Input: dimensioned drawing with shaded views. Units: mm. Origin: part minimum x, y, z. A direction names the side the tool comes from. Coordinates: 2 decimals unless noted, no trailing zeros. Write each loop counter-clockwise with the first axis right and the second up, starting at its lowest first coordinate (ties: lowest second). Pieces come first, ordered by that corner, then holes. Notation, with made-up numbers: M 19.5,68 L 49.5,68 A13 ccw 49.5,93 Z; hole C 23,19 d7. An arc over 180 degrees is marked long. Use one line per item in the form item = value.
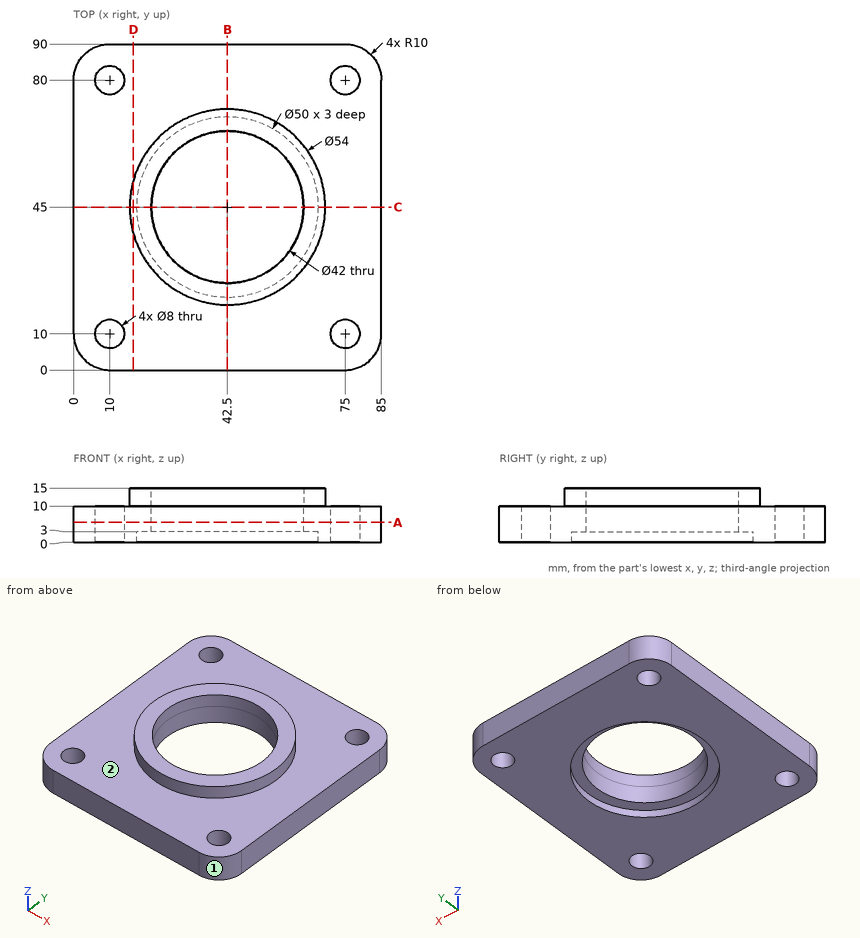
(1) Section query C-C on y = 45. Return the cut outline in (x, z), plus the area to 3 significant figures.
Computed:
outline = M 0,0 L 17.5,0 L 17.5,3 L 21.5,3 L 21.5,15 L 15.5,15 L 15.5,10 L 0,10 Z; M 63.5,3 L 67.5,3 L 67.5,0 L 85,0 L 85,10 L 69.5,10 L 69.5,15 L 63.5,15 Z
area = 466 mm^2
(2) Section query A-A on z = 5.5. Return the cut outline in (x, y), plus the area to 3 significant figures.
Computed:
outline = M 0,10 A10 ccw 10,0 L 75,0 A10 ccw 85,10 L 85,80 A10 ccw 75,90 L 10,90 A10 ccw 0,80 Z; hole C 10,10 d8; hole C 10,80 d8; hole C 42.5,45 d42; hole C 75,10 d8; hole C 75,80 d8
area = 5,980 mm^2
(3) Set-up query: the marked faces 1 and 2. Return all of +Z, -Z, +X, -X, +Y, -Y with unobstructed straight access to the full face (end or side cutting, diameter ignored); none if empty.
Computed:
face_1 = +Z, -Z, +X, -Y
face_2 = +Z
(4) Section query B-B on x = 42.5. Return the cut outline in (y, z), plus the area to 3 significant figures.
Computed:
outline = M 0,0 L 20,0 L 20,3 L 24,3 L 24,15 L 18,15 L 18,10 L 0,10 Z; M 66,3 L 70,3 L 70,0 L 90,0 L 90,10 L 72,10 L 72,15 L 66,15 Z
area = 516 mm^2
(5) First-contact query: pin 1 Ø1.5 at (x, z) = (20, 12) entering from +Y; pin 2 Ø1 at (x, z) = (64.5, 12) entering from -Y. Flat tips, straight axial feed; report the tip coordinate or a pass-through.
Computed:
pin_1 = 61
pin_2 = 28.67
(6) Section query D-D on x = 16.5. Return the cut outline in (y, z), plus the area to 3 significant figures.
Computed:
outline = M 0,0 L 90,0 L 90,10 L 52.28,10 L 52.28,15 L 37.72,15 L 37.72,10 L 0,10 Z
area = 973 mm^2
(7) Line query: probe 1 along Y at (x, z) = (75, 4); probe 2 along Y at (x, z) = (42.5, 6.75); probe 3 along X at (y, z) = (45, 1.95). Output: solid intervals per line, ascending.
Computed:
probe_1 = 0 to 6, 14 to 76, 84 to 90
probe_2 = 0 to 24, 66 to 90
probe_3 = 0 to 17.5, 67.5 to 85
